CAD build for the part. Positions are in the model's coordinates, mm. Give positions to 0.01 mm unless a question says otherwise; leave off trailing zeros. Loops run counter-clockwise (first coordinate to the right, second up) from the corner with the lowest first, then second, coordinate; pieces in that order, holes last.
```python
from build123d import *

# Parameters (mm, degrees)
BOSS_EXTRUDE1_DEPTH = 1.5875


with BuildPart() as part:
    # Sketch1 → Boss-Extrude1 (new, symmetric)
    with BuildSketch(Plane(origin=(0, 0, 0), x_dir=(1, 0, 0), z_dir=(0, 1, 0))):
        with BuildLine():
            Line((1020.4196, -520.7), (1020.4196, -384.668661408))
            Line((1020.4196, -384.668661408), (1017.2446, -384.668661408))
            Line((1017.2446, -384.668661408), (814.0446, -384.668661408))
            Line((814.0446, -384.668661408), (814.0446, -419.1))
            Line((814.0446, -419.1), (525.1196, -419.1))
            Line((525.1196, -419.1), (521.9446, -419.1))
            Line((521.9446, -419.1), (521.9446, -520.7))
            Line((521.9446, -520.7), (525.1196, -520.7))
            Line((525.1196, -520.7), (893.2418, -520.7))
            ThreePointArc((893.2418, -520.7), (906.3228, -507.619), (919.4038, -520.7))
            Line((919.4038, -520.7), (1020.4196, -520.7))
        make_face()
    extrude(amount=BOSS_EXTRUDE1_DEPTH, both=True)


solid = part.part
```
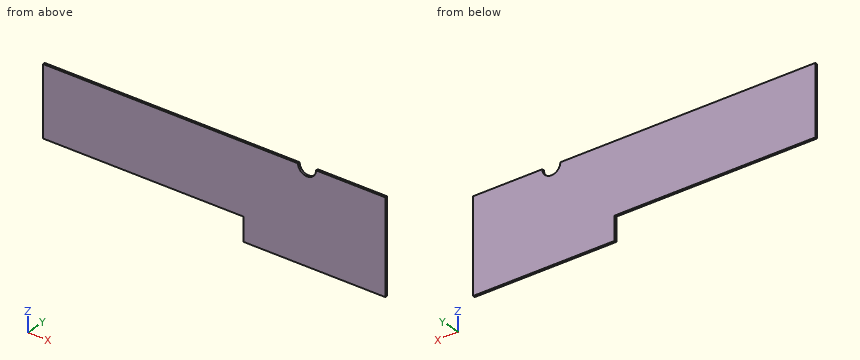
1. Drop a flat-ended pin along its axis: pin 1 (1.6 mm diameter, centred on x = 597.5, y = -0.5, fed in from -Z). Give the stop position or say it passes through.
Responses:
pin 1: stops at z = 419.1
2. Probe line 1 along Z through (x, y) = (553, 1.05); line 2 along X through (y, z) = (0.1, 401); line 3 along Z through (x, y) = (898, 0.7). List the from-to ranges inside material, lowest first.
Responses:
line 1: z = 419.1 to 520.7
line 2: x = 814.04 to 1020.42
line 3: z = 384.67 to 510.61
3. Saw through at B-B, the plane x = 795. List the corners of the cut face in (y, z), and give its area (3 significant figures).
Responses:
outline: (-1.59, 419.1) - (1.59, 419.1) - (1.59, 520.7) - (-1.59, 520.7) - close
area: 323 mm2
4. Saw through at A-A, the plane y = 0.4. List the corners of the cut face in (x, z).
Responses:
outline: (521.94, 419.1) - (814.04, 419.1) - (814.04, 384.67) - (1020.42, 384.67) - (1020.42, 520.7) - (919.4, 520.7) arc R13.08 cw to (893.24, 520.7) - (521.94, 520.7) - close
5. Saw through at C-C, the plane z = 404.5. List the corners of the cut face in (x, y), and give its area (3 significant figures).
Responses:
outline: (814.04, -1.59) - (1020.42, -1.59) - (1020.42, 1.59) - (814.04, 1.59) - close
area: 655 mm2
